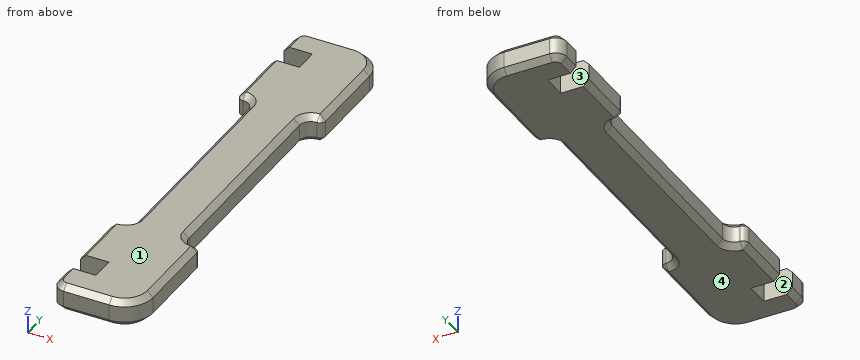
Autodesk Fusion 360 part; units mm, degrees
sketch "Sketch1" plane through (0, 0, 0) normal (0, 0, 1) x (1, 0, 0)
  line L0 (7.5, -40.2) -> (-7.5, -40.2)
  line L1 (-7.5, -40.2) -> (-7.5, 40.2)
  line L2 (-7.5, 40.2) -> (7.5, 40.2)
  line L3 (7.5, 40.2) -> (7.5, -40.2)
  line L4 (7.5, -40.2) -> (-7.5, 40.2) construction
  line L5 (-7.5, -40.2) -> (7.5, 40.2) construction
  line L6 (-7.5, 35.2) -> (-2.5, 35.2)
  line L7 (-2.5, 35.2) -> (-2.5, 31)
  line L8 (-2.5, 31) -> (-7.5, 31)
  line L9 (-7.5, 31) -> (-7.5, 35.2)
  line L10 (-7.5, -31) -> (-2.5, -31)
  line L11 (-2.5, -31) -> (-2.5, -35.2)
  line L12 (-2.5, -35.2) -> (-7.5, -35.2)
  line L13 (-7.5, -35.2) -> (-7.5, -31)
  line L14 (0, 1.75) -> (0, 22.5)
  line L15 (-7.5, 20) -> (-4.5, 20)
  line L16 (-4.5, 20) -> (-4.5, -20)
  line L17 (-4.5, -20) -> (-7.5, -20)
  line L18 (-7.5, -20) -> (-7.5, 20)
  line L19 (7.5, -20) -> (4.5, -20)
  line L20 (4.5, -20) -> (4.5, 20)
  line L21 (4.5, 20) -> (7.5, 20)
  line L22 (7.5, 20) -> (7.5, -20)
  dimension "d1" = 80.4
  dimension "d2" = 15
  dimension "d3" = 5
  dimension "d4" = 4.2
  dimension "d5" = 5
  dimension "d6" = 4.2
  dimension "d7" = 5
  dimension "d8" = 5
  dimension "d26" = 15
  dimension "d27" = 40.2
  dimension "d28" = 3
  dimension "d29" = 40
  dimension "d30" = 20
  dimension "d31" = 40
  dimension "d32" = 3
  dimension "d33" = 20
extrude "Extrude1" add sketch "Sketch1" along normal blind 4.8 contours L0 L1 L2 L3 L6 L7 L8 L10 L11 L12 L15 L16 L17 L19 L20 L21
fillet "Fillet1" radius 5 2 edges at (7.5, 40.2, 2.4) (7.5, -40.2, 2.4)
fillet "Fillet1" radius 2 6 edges at (-7.5, 40.2, 2.4) (-7.5, -40.2, 2.4) (-4.5, 20, 2.4) (4.5, 20, 2.4) (4.5, -20, 2.4) (-4.5, -20, 2.4)
fillet "Fillet1" radius 1 4 edges at (-7.5, 20, 2.4) (7.5, 20, 2.4) (-7.5, -20, 2.4) (7.5, -20, 2.4)
chamfer "Chamfer1" distance 1 angle 45 44 edges at (7.5, 28.1, 4.8) (7.2071, 20.2929, 4.8) (5.0858, 19.4142, 4.8) (4.5, 0, 4.8) (5.0858, -19.4142, 4.8) (7.2071, -20.2929, 4.8) (7.5, -28.1, 4.8) (6.0355, -38.7355, 4.8) (-1.5, -40.2, 4.8) (-6.9142, -39.6142, 4.8) (-7.5, -36.7, 4.8) (-7.5, 36.7, 4.8) (-6.9142, 39.6142, 4.8) (-1.5, 40.2, 4.8) (6.0355, 38.7355, 4.8) (7.5, -28.1, 0) (7.2071, -20.2929, 0) (5.0858, -19.4142, 0) (4.5, 0, 0) (5.0858, 19.4142, 0) (7.2071, 20.2929, 0) (7.5, 28.1, 0) (6.0355, 38.7355, 0) (-1.5, 40.2, 0) (-6.9142, 39.6142, 0) (-7.5, 36.7, 0) (-7.5, -36.7, 0) (-6.9142, -39.6142, 0) (-1.5, -40.2, 0) (6.0355, -38.7355, 0) (-7.5, -26, 0) (-7.2071, -20.2929, 0) (-5.0858, -19.4142, 0) (-4.5, 0, 0) (-5.0858, 19.4142, 0) (-7.2071, 20.2929, 0) (-7.5, 26, 0) (-7.5, 26, 4.8) (-7.2071, 20.2929, 4.8) (-5.0858, 19.4142, 4.8) (-4.5, 0, 4.8) (-5.0858, -19.4142, 4.8) (-7.2071, -20.2929, 4.8) (-7.5, -26, 4.8)
equation "d27 = d1 / 2"
equation "d30 = d29 / 2"
equation "d33 = d31 / 2"
Design review of the part built by this model. Coordinates are the model's own, in mm. Face numbers are marked on the shaded views. A direction names the side the tool comes from. Coordinates: 2 decimals unless noted, no trailing zeros. Order: outer loops, then holes, each group sorted by start corner. A loop starts at its lowest first (then second) coordinate and runs counter-clockwise, first axis right, second up. Notation, with made-up numbers: M 64.25,37 L 108.25,37 A17 ccw 108.25,45 Z; hole C 13,-29 d10. An arc over 180 degrees is marked long. Use a Markdown table: item, result.
(1) Add section A-A (y = 12.5). Give the boundary of the cut face in (x, z), then the cut area to 3 significant figures.
Worked answers:
| item | result |
|---|---|
| outline | M -4.5,1 L -3.5,0 L 3.5,0 L 4.5,1 L 4.5,3.8 L 3.5,4.8 L -3.5,4.8 L -4.5,3.8 Z |
| area | 41.2 mm2 |
(2) Wall thickness on probe 1 along Y at (x, z) = (-4.25, 3); probe 2 along Y at (x, z) = (-4, 3.85); probe 3 along X at (y, z) = (-35.5, 3.1): over which ranges is each line inside the solid? List them lowest first.
Worked answers:
| item | result |
|---|---|
| probe 1 | y = -40.2 to -35.2, -31 to 31, 35.2 to 40.2 |
| probe 2 | y = -40.15 to -35.2, -31 to 31, 35.2 to 40.15 |
| probe 3 | x = -7.5 to 7.49 |
(3) Add section C-C (y = -25). Give the boundary of the cut face in (x, z), then the cut area to 3 significant figures.
Worked answers:
| item | result |
|---|---|
| outline | M -7.5,1 L -6.5,0 L 6.5,0 L 7.5,1 L 7.5,3.8 L 6.5,4.8 L -6.5,4.8 L -7.5,3.8 Z |
| area | 70.0 mm2 |
(4) Draft analysis for pull direction Y (two halves, no side actions). For the marked faces 3 and 4, state which applies: released by +Y, released by -Y, zero draft, split by the parting line, or undercut.
Worked answers:
| item | result |
|---|---|
| face 3 | undercut |
| face 4 | zero draft |
(5) For P1, Ø1.3, axis at y = 33, z = 1.5, coming from the -X side, flat-tipped, find the tip position at first contact; note if it passes through.
Worked answers:
| item | result |
|---|---|
| P1 | stops at x = -2.5 |
(6) For the marked faces 1 and 2, list the 3-axis set-ups (+Z, -Z, +X, -X, +Y, -Y) from which the entire face can be reached by the end or side of a thin tool; tool diameter is ignored.
Worked answers:
| item | result |
|---|---|
| face 1 | +Z, +X, -X, +Y, -Y |
| face 2 | +Z, -Z, -X |
